Autodesk Inventor part; units mm, degrees
ref_plane "CP_XY" through (0, 6.6, 0) normal (0, 0, 1) x (1, 0, 0)
ref_plane "CP_YZ" through (0, 6.6, 0) normal (1, 0, 0) x (0, 1, 0)
ref_plane "CP_ZX" through (0, 6.6, 0) normal (0, 1, 0) x (0, 0, 1)
sketch "Sketch_1" plane through (0, 0, 0) normal (1, 0, 0) x (0, 1, 0)
  line L0 (6.6, 0) -> (0.379, -1.5511)
  arc A0 (0.379, -1.5511) -> (0, -2.0362) centre (0.5, -2.0362) ccw
  line L1 (0, -2.0362) -> (0, -36.1119)
  arc A1 (0, -36.1119) -> (0.6316, -37.7729) centre (2.5, -36.1119) ccw
  arc A2 (0.6316, -37.7729) -> (5.0923, -40.9212) centre (9.6, -29.8) ccw
  arc A3 (5.0923, -40.9212) -> (5.3576, -40.7976) centre (5.1674, -40.7358) ccw
  line L2 (5.3576, -40.7976) -> (5.9417, -39)
  line L3 (5.9417, -39) -> (6.6, -39)
  line L4 (6.6, -39) -> (6.6, 0)
extrude "Extrusion1" add sketch "Sketch_1" along normal mid plane 12.5
sketch "Sketch_2" plane through (0, 0, 0) normal (1, 0, 0) x (0, 1, 0)
  line L0 (6.6, -1.5459) -> (1.879, -2.723)
  arc A0 (1.879, -2.723) -> (1.5, -3.2081) centre (2, -3.2081) ccw
  line L1 (1.5, -3.2081) -> (1.5, -35.8)
  line L2 (1.5, -35.8) -> (6.6, -35.8)
  line L3 (6.6, -35.8) -> (6.6, -1.5459)
extrude "Extrusion2" cut sketch "Sketch_2" along normal mid plane 8.2
sketch "Sketch_3" plane through (6.25, 0, 0) normal (1, 0, 0) x (0, 0, -1)
  line L0 (32.75, 6.6) -> (42, 0.1231)
  line L1 (42, 0.1231) -> (42, 6.6)
  line L2 (42, 6.6) -> (32.75, 6.6)
extrude "Extrusion3" cut sketch "Sketch_3" against normal blind 1
sketch "Sketch_4" plane through (-6.25, 0, 0) normal (1, 0, 0) x (0, 0, -1)
  line L0 (32.75, 6.6) -> (42, 0.1231)
  line L1 (42, 0.1231) -> (42, 6.6)
  line L2 (42, 6.6) -> (32.75, 6.6)
extrude "Extrusion4" cut sketch "Sketch_4" along normal blind 1
sketch "Sketch_5" plane through (0, 0, 0) normal (1, 0, 0) x (0, 1, 0)
  line L0 (6.6, -38.32) -> (0, -38.32)
  line L1 (0, -38.32) -> (0, -42)
  line L2 (0, -42) -> (6.6, -42)
  line L3 (6.6, -42) -> (6.6, -38.32)
extrude "Extrusion5" cut sketch "Sketch_5" along normal mid plane 4.2
ref_plane "CP_XY" through (0, 6.6, 0) normal (0, 0, 1) x (1, 0, 0)
ref_plane "CP_YZ" through (0, 6.6, 0) normal (1, 0, 0) x (0, 1, 0)
ref_plane "CP_ZX" through (0, 6.6, 0) normal (0, 1, 0) x (0, 0, 1)
properties part number "CH20M LF OR 1103640000"
CAD build for the part. Positions are in the model's coordinates, mm. A direction names the side the tool comes from. Coordinates: 2 decimals unless noted, no trailing zeros. Loops run counter-clockwise (first coordinate to the right, second up) from the corner with the lowest first, then second, coordinate; pieces in that order, holes last. Notation, with made-up numbers: (0.25, 23) -> (16.25, 23) arc R28 ccw to (16.25, 49) -> close; hole circle Ø4 at (80, 78). An arc over 180 degrees is marked (long way). One line per item, written item: value.
1. Slice it at C-C on z = -13. Write the cut outline in (x, y).
Answers:
outline: (-6.25, 0) -> (6.25, 0) -> (6.25, 6.6) -> (4.1, 6.6) -> (4.1, 1.5) -> (-4.1, 1.5) -> (-4.1, 6.6) -> (-6.25, 6.6) -> close
2. Slice it at D-D on x = -3.5. Write the cut outline in (y, z).
Answers:
outline: (0, -36.11) arc R2.5 ccw to (0.63, -37.77) arc R12 ccw to (5.09, -40.92) arc R0.2 ccw to (5.36, -40.8) -> (5.94, -39) -> (6.6, -39) -> (6.6, -35.8) -> (1.5, -35.8) -> (1.5, -3.21) arc R0.5 cw to (1.88, -2.72) -> (6.6, -1.55) -> (6.6, 0) -> (0.38, -1.55) arc R0.5 ccw to (0, -2.04) -> close
3. Drill centre lines: line 1 (X direction, y = 4.5, z = -35.5); line 2 (Z direction, x = -1.25, y = 3.5); line 3 (Y direction, x = 1, z = -11). Where is each one in solid material? Low to high. Write a range as [from, to].
Answers:
line 1: x = [-6.25, -4.1], [4.1, 6.25]
line 2: z = [-38.32, -35.8], [-2.32, -0.77]
line 3: y = [0, 1.5]
4. Which spindle directions (+Z, -Z, +X, -X, +Y, -Y) get a long thin tool onto all of the face, cutting with end or side? Do faces 5 (the face through (-0.057, 4.273, -2.126)), 6 (the face through (-5.76, 4.38, -35.92)), 7 (the face through (-2.1, 4, -39)), 8 (the face through (5.76, 4.38, -35.92)). Say none if no direction does.
Answers:
face 5: +Y
face 6: -Z, -X, +Y
face 7: -Z, +Y, -Y
face 8: -Z, +X, +Y
5. Flat gauge pins, fed straight in: P1, Ø2, axis at x = -0.5, y = 5, coming from the -Z side; P2, Ø5, axis at x = 3.5, z = -28.5, coming from the +Y side; P3, Ø3, axis at x = -2, y = 3, coming from the +Z side; P4, Ø0.7, axis at x = -4, y = 6.5, coming from the -Z side. Where does each tip first touch, or does it go through?
Answers:
P1: stops at z = -38.32
P2: stops at y = 6.6
P3: stops at z = -0.52
P4: stops at z = -39
6. Pull direction X, two halves, no side cores. Call faces 1 (the face through (0, 0, -19)), 2 (the face through (4.1, 4, -18)), 3 (the face through (2.1, 4, -39)), 4 (the face through (-6.25, 3, -19)): pulls with the +X half, pulls with the -X half, needs draft (parallel to the pull), parting line crosses it, or undercut.
Answers:
face 1: needs draft
face 2: undercut
face 3: undercut
face 4: pulls with the -X half
7. Slice it at A-A on x = -0.25. Write the cut outline in (y, z), and give its area (3 significant figures).
Answers:
outline: (0, -36.11) arc R2.5 ccw to (0.63, -37.77) arc R12 ccw to (1.15, -38.32) -> (6.6, -38.32) -> (6.6, -35.8) -> (1.5, -35.8) -> (1.5, -3.21) arc R0.5 cw to (1.88, -2.72) -> (6.6, -1.55) -> (6.6, 0) -> (0.38, -1.55) arc R0.5 ccw to (0, -2.04) -> close
area: 75.2 mm^2
8. Slice it at B-B on y = 4.25. Write the cut outline in (x, z), and give its area (3 significant figures).
Answers:
outline: (-6.25, -36.11) -> (-5.25, -36.11) -> (-5.25, -40.54) -> (-2.1, -40.54) -> (-2.1, -38.32) -> (2.1, -38.32) -> (2.1, -40.54) -> (5.25, -40.54) -> (5.25, -36.11) -> (6.25, -36.11) -> (6.25, -0.59) -> (-6.25, -0.59) -> close; hole (-4.1, -35.8) -> (4.1, -35.8) -> (4.1, -2.13) -> (-4.1, -2.13) -> close
area: 205 mm^2
